Autodesk Inventor part; units mm, degrees
ref_plane "YZ Plane" through (0, 0, 0) normal (1, 0, 0) x (0, 1, 0)
ref_plane "XZ Plane" through (0, 0, 0) normal (0, 1, 0) x (-1, 0, 0)
ref_plane "XY Plane" through (0, 0, 0) normal (0, 0, 1) x (1, 0, 0)
sketch "Sketch1" plane through (0, 0, 0) normal (0, 0, 1) x (1, 0, 0)
  line L0 (-89, 89) -> (89, 89)
  line L1 (89, 89) -> (89, -89)
  line L2 (89, -89) -> (-89, -89)
  line L3 (-89, -89) -> (-89, 89)
  line L4 (-78.5, 42.5) -> (-74, 42.5)
  line L5 (-74, 42.5) -> (-74, -42.5)
  line L6 (-74, -42.5) -> (-78.5, -42.5)
  line L7 (42.5, 78.5) -> (42.5, 74)
  line L8 (42.5, 74) -> (-42.5, 74)
  line L9 (-42.5, 74) -> (-42.5, 78.5)
  line L10 (78.5, 42.5) -> (74, 42.5)
  line L11 (74, 42.5) -> (74, -42.5)
  line L12 (74, -42.5) -> (78.5, -42.5)
  line L13 (42.5, -78.5) -> (42.5, -74)
  line L14 (42.5, -74) -> (-42.5, -74)
  line L15 (-42.5, -74) -> (-42.5, -78.5)
  line L16 (-78.5, 78.5) -> (-42.5, 78.5)
  line L17 (42.5, 78.5) -> (78.5, 78.5)
  line L18 (-78.5, -78.5) -> (-78.5, -42.5)
  line L19 (-78.5, 42.5) -> (-78.5, 78.5)
  line L20 (78.5, -78.5) -> (42.5, -78.5)
  line L21 (-42.5, -78.5) -> (-78.5, -78.5)
  line L22 (78.5, 78.5) -> (78.5, 42.5)
  line L23 (78.5, -42.5) -> (78.5, -78.5)
  point P0 (0, 0)
  point P1 (-74, 0)
  point P2 (0, 74)
  dimension "d0" = 36
  dimension "d1" = 36
  dimension "d2" = 148
  dimension "d3" = 148
  dimension "d4" = 157
  dimension "d5" = 157
  dimension "d6" = 74
  dimension "d7" = 74
  dimension "d9" = 15
  dimension "d14" = 15
  dimension "d15" = 15
extrude "Extrusion1" add sketch "Sketch1" along normal blind 5
sketch "Sketch2" plane through (0, 0, 5) normal (0, 0, 1) x (1, 0, 0)
  circle A0 centre (-81.5, 0) radius 2
  circle A1 centre (81.5, 0) radius 2
  line L0 (-74, -42.5) -> (-74, 42.5)
  line L1 (74, 42.5) -> (74, -42.5)
  circle A2 centre (0, 81.5) radius 2
  circle A3 centre (0, -81.5) radius 2
  line L2 (-42.5, 74) -> (42.5, 74)
  line L3 (42.5, -74) -> (-42.5, -74)
  point P0 (0, 0)
  dimension "d16" = 7.5
  dimension "d17" = 7.5
  dimension "d18" = 4
  dimension "d19" = 7.5
  dimension "d20" = 7.5
hole "Hole1" at (-81.5, 0, 5) at (0, 81.5, 5) at (81.5, 0, 5) at (0, -81.5, 5) direction (0, 0, -1) diameter 4 end through all
fillet "Fillet1" radius 2 4 edges at (-89, -89, 2.5) (-89, 89, 2.5) (89, -89, 2.5) (89, 89, 2.5)
equation "\"d21\" = d18"
properties part number "WaagePlexiMittelsteuck" material "PET Plastic"
Could you check a few things on this model? Use its own coordinates, in mm. A direction names the side the tool comes from. Round coordinates to 2 decimals unless told otherwise and drop trailing zeros. Loops run counter-clockwise (first coordinate to the right, second up) from the corner with the lowest first, then second, coordinate; pieces in that order, holes last. Notation, with made-up numbers: M 66.5,42 L 109.5,42 A19 cw 109.5,70 Z; hole C -25,84.25 d6. An arc over 180 degrees is marked long. Answer as CSV lines item,"result".
1) Which directions (+Z, -Z, +X, -X, +Y, -Y) give clear straight access to the entire face, cutting with the end or side of a thin tool? Please do faces 1 (the flat face through (89, 1, 2)), 2 (the flat face through (1, -74, 2)).
From the geometry:
face 1,"+Z, -Z, +X, +Y, -Y"
face 2,"+Z, -Z"
2) Imagine slicing it at A-A on x = 30. List the corners of the cut face in (y, z) for me, and give its area (3 significant figures).
From the geometry:
outline,"M -89,0 L -74,0 L -74,5 L -89,5 Z; M 74,0 L 89,0 L 89,5 L 74,5 Z"
area,"150 mm^2"
3) Imagine slicing it at C-C on z = 1.65. Count the separate pieces of the cut face and the enclosed holes in it, and give its area (3 significant figures).
From the geometry:
separate pieces,"1"
enclosed holes,"5"
area,"8,510 mm^2"
4) If I drill on probe 1 along Y at (x, z) = (76.5, 0.85); probe 2 along X at (y, z) = (0, 1.55), over which ranges is the centre line in solid material (lowest first)?
From the geometry:
probe 1,"-89 to -78.5, -42.5 to 42.5, 78.5 to 89"
probe 2,"-89 to -83.5, -79.5 to -74, 74 to 79.5, 83.5 to 89"
